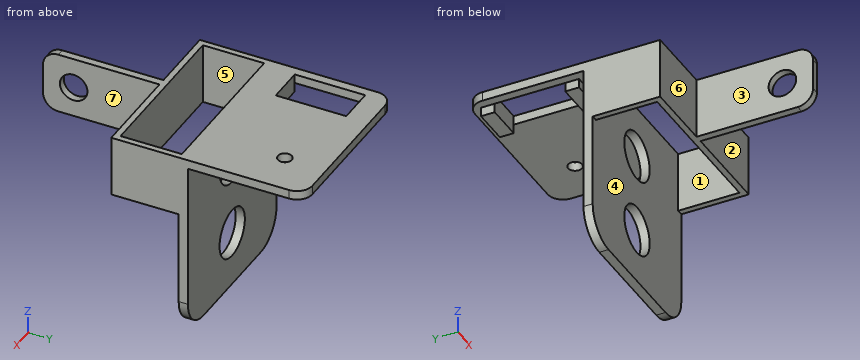
from build123d import *

# Parameters (mm, degrees)
SKETCH1_W                = 50
SKETCH1_H                = 57.8
BOSS_EXTRUDE1_DEPTH      = 3
SKETCH1_3_W              = 50
SKETCH1_3_H              = 3
BOSS_EXTRUDE2_DEPTH      = 63
SKETCH7_W                = 10
SKETCH7_H                = 20
BOSS_EXTRUDE6_DEPTH      = 60
SKETCH8_W                = 7.5
SKETCH8_H                = 20
CUT_EXTRUDE4_DEPTH       = 60
SKETCH10_R               = 4.5
CUT_EXTRUDE5_DEPTH       = 60
FILLET1_R                = 5
FILLET2_R                = 5
CUT_EXTRUDE6_REACH       = 93.771
FILLET4_R                = 5
BOSS_EXTRUDE7_DEPTH      = 3
BOSS_EXTRUDE8_DEPTH      = 3
SKETCH15_R               = 8
CUT_EXTRUDE7_DEPTH       = 3
CUT_EXTRUDE8_DEPTH       = 40
BOSS_EXTRUDE9_DEPTH      = 23
BOSS_EXTRUDE9_DEPTH_BACK = 33
SKETCH17_W               = 20
SKETCH17_H               = 2
BOSS_EXTRUDE25_REACH     = 95.87
SKETCH19_W               = 54
SKETCH19_H               = 20
SKETCH19_W_2             = 2
CUT_EXTRUDE9_REACH       = 83.018
CUT_EXTRUDE10_REACH      = 78.756
SKETCH27_R               = 8
SKETCH28_W               = 12
SKETCH28_H               = 4.5
BOSS_EXTRUDE26_DEPTH     = 3
SKETCH28_3_W             = 12
SKETCH28_3_H             = 23
CUT_EXTRUDE11_DEPTH      = 3
SKETCH29_W               = 56
SKETCH29_H               = 22
CUT_EXTRUDE12_DEPTH      = 3
FILLET5_R                = 5
FILLET6_R                = 10
CUT_EXTRUDE13_REACH      = 90.719
SKETCH30_R               = 2.271159968


with BuildPart() as part:
    # Sketch1 → Boss-Extrude1 (new body)
    with BuildSketch(Plane(origin=(0, 0, 0), x_dir=(1, 0, 0), z_dir=(0, 1, 0))):
        with Locations((2.5, 0.4)):
            Rectangle(SKETCH1_W, SKETCH1_H)
    extrude(amount=BOSS_EXTRUDE1_DEPTH)

    # Sketch1<3> → Boss-Extrude2 (add)
    with BuildSketch(Plane(origin=(0, 0, 0), x_dir=(1, 0, 0), z_dir=(0, 1, 0))):
        with Locations((2.5, -30)):
            Rectangle(SKETCH1_3_W, SKETCH1_3_H)
    extrude(amount=BOSS_EXTRUDE2_DEPTH)

    # Sketch7 → Boss-Extrude6 (add)
    with BuildSketch(Plane.XZ):
        with Locations((2.5, 21.5)):
            Rectangle(SKETCH7_W, SKETCH7_H)
    extrude(amount=BOSS_EXTRUDE6_DEPTH)

    # Sketch8 → Cut-Extrude4 (cut)
    with BuildSketch(Plane(origin=(0, 0, 11.5), x_dir=(-1, 0, 0), z_dir=(0, 0, -1))):
        with Locations((-3.75, -50)):
            Rectangle(SKETCH8_W, SKETCH8_H)
    extrude(amount=-CUT_EXTRUDE4_DEPTH, mode=Mode.SUBTRACT)

    # Sketch10 → Cut-Extrude5 (cut)
    with BuildSketch(Plane(origin=(0, 0, 0), x_dir=(0, 0, -1), z_dir=(1, 0, 0))):
        with Locations((-21.5, -50)):
            Circle(SKETCH10_R)
    extrude(amount=-CUT_EXTRUDE5_DEPTH, mode=Mode.SUBTRACT)

    # Fillet1
    fillet1_edges = [part.edges().sort_by_distance(p)[0] for p in [
        (7.5, -20, 11.5),
    ]]
    fillet(fillet1_edges, radius=FILLET1_R)

    # Fillet2
    fillet2_edges = [part.edges().sort_by_distance(p)[0] for p in [
        (7.5, -20, 31.5),
    ]]
    fillet(fillet2_edges, radius=FILLET2_R)

    # Sketch11 → Cut-Extrude6 (cut, up to next)
    with BuildSketch(Plane.XY.offset(31.5), mode=Mode.PRIVATE) as cut_extrude6_sk1:
        with BuildLine():
            Line((7.5, -40), (0, -40))
            Line((0, -40), (0, -20))
            ThreePointArc((0, -20), (2.621852946, -15.723111223), (7.5, -14.552824164))
            Line((7.5, -14.552824164), (7.5, -40))
        make_face()
    cut_extrude6_tool1 = extrude(cut_extrude6_sk1.sketch, amount=-CUT_EXTRUDE6_REACH, mode=Mode.PRIVATE) & part.part
    add(cut_extrude6_tool1.solids().sort_by_distance((3.859065, -27.782641, 31.5))[0], mode=Mode.SUBTRACT)

    # Fillet4
    fillet4_edges = [part.edges().sort_by_distance(p)[0] for p in [
        (-1.25, -60, 11.5),
        (-1.25, -60, 31.5),
    ]]
    fillet(fillet4_edges, radius=FILLET4_R)

    # Sketch13 → Boss-Extrude7 (add)
    with BuildSketch(Plane(origin=(27.5, 0, 0), x_dir=(0, 0, -1), z_dir=(1, 0, 0))):
        Polygon((-31.5, 0), (29.3, 0), (29.3, 3), (-28.5, 3), (-28.5, 63), (-31.5, 63), align=None)
    extrude(amount=BOSS_EXTRUDE7_DEPTH)

    # Sketch14 → Boss-Extrude8 (add)
    with BuildSketch(Plane.ZY.offset(22.5)):
        Polygon((-29.3, 0), (31.5, 0), (31.5, 63), (28.5, 63), (28.5, 3), (-29.3, 3), align=None)
    extrude(amount=BOSS_EXTRUDE8_DEPTH)

    # Sketch15 → Cut-Extrude7 (cut)
    with BuildSketch(Plane(origin=(0, 3, 0), x_dir=(1, 0, 0), z_dir=(0, 1, 0))):
        with Locations(Location((2.5, 11.3, 0), (0, 0, 270))):
            Circle(SKETCH15_R)
        with Locations(Location((2.5, -14.7, 0), (0, 0, 270))):
            Circle(SKETCH15_R)
    extrude(amount=-CUT_EXTRUDE7_DEPTH, mode=Mode.SUBTRACT)

    # Sketch16 → Cut-Extrude8 (cut, symmetric)
    with BuildSketch(Plane(origin=(0, 0, 0), x_dir=(0, 0, -1), z_dir=(1, 0, 0))):
        Polygon((-31.5, -20), (-11.5, -20), (-11.5, 0), (-31.5, 0.262000387), align=None)
    extrude(amount=CUT_EXTRUDE8_DEPTH, both=True, mode=Mode.SUBTRACT)


with BuildPart() as cut_extrude8_piece_1:
    # of the separate pieces the step leaves, piece 1, a body of its own (cut_extrude8_pieces)
    add(part.part.solids().sort_by_distance((30.5, 63, 31.5))[0])



with BuildPart() as cut_extrude8_piece_2:
    # of the separate pieces the step leaves, piece 2, a body of its own (cut_extrude8_pieces)
    add(part.part.solids().sort_by_distance((0, -55, 31.5))[0])

    # Sketch17 → Boss-Extrude9 (add, two sides: drawn at the far end of the back side and taken through both)
    with BuildSketch(Plane.ZY.offset(2.5).offset(-BOSS_EXTRUDE9_DEPTH_BACK)):
        with Locations((21.5, -21)):
            Rectangle(SKETCH17_W, SKETCH17_H)
    extrude(amount=BOSS_EXTRUDE9_DEPTH + BOSS_EXTRUDE9_DEPTH_BACK)


with BuildPart() as cut_extrude8_piece_1_1:
    add(cut_extrude8_piece_1.part)

    add(cut_extrude8_piece_2.part)  # Boss-Extrude25 merges Cut-Extrude8 piece 2
    # Boss-Extrude25: up to this plane
    boss_extrude25_end = Plane(origin=(-40, 0, 11.5), z_dir=(0, 0.9999142057885084, -0.013098895462462855))
    # Sketch19 → Boss-Extrude25 (add, up to the surface)
    with BuildSketch(Plane(origin=(0, -20, 0), x_dir=(1, 0, 0), z_dir=(0, 1, 0)), mode=Mode.PRIVATE) as boss_extrude25_sk1:
        with Locations((1.5, -21.5)):
            Rectangle(SKETCH19_W, SKETCH19_H)
    boss_extrude25_tool1 = split(extrude(boss_extrude25_sk1.sketch, amount=BOSS_EXTRUDE25_REACH, mode=Mode.PRIVATE), bisect_by=boss_extrude25_end, keep=Keep.BOTH, mode=Mode.PRIVATE)
    add(boss_extrude25_tool1.solids().sort_by_distance((1.5, -20, 21.5))[0])
    # Sketch19 → Boss-Extrude25 (add, up to the surface)
    with BuildSketch(Plane(origin=(0, -20, 0), x_dir=(1, 0, 0), z_dir=(0, 1, 0)), mode=Mode.PRIVATE) as boss_extrude25_sk2:
        with Locations((29.5, -21.5)):
            Rectangle(SKETCH19_W_2, SKETCH19_H)
    boss_extrude25_tool2 = split(extrude(boss_extrude25_sk2.sketch, amount=BOSS_EXTRUDE25_REACH, mode=Mode.PRIVATE), bisect_by=boss_extrude25_end, keep=Keep.BOTH, mode=Mode.PRIVATE)
    add(boss_extrude25_tool2.solids().sort_by_distance((29.5, -20, 21.5))[0])

    # Sketch25 → Cut-Extrude9 (cut, up to next)
    with BuildSketch(Plane(origin=(0, 0, 11.5), x_dir=(-1, 0, 0), z_dir=(0, 0, -1)), mode=Mode.PRIVATE) as cut_extrude9_sk1:
        Polygon((-9.832121112, 0), (-28.5, 0), (-28.5, -20), (23.5, -20), (23.5, 0), (4.832121112, 0), align=None)
    cut_extrude9_tool1 = extrude(cut_extrude9_sk1.sketch, amount=-CUT_EXTRUDE9_REACH, mode=Mode.PRIVATE) & cut_extrude8_piece_1_1.part
    add(cut_extrude9_tool1.solids().sort_by_distance((2.5, -10, 11.5))[0], mode=Mode.SUBTRACT)

    # Sketch27 → Cut-Extrude10 (cut, up to next)
    with BuildSketch(Plane.XZ, mode=Mode.PRIVATE) as cut_extrude10_sk1:
        with Locations(Location((2.5, 14.7, 0), (0, 0, 90))):
            Circle(SKETCH27_R)
    cut_extrude10_tool1 = extrude(cut_extrude10_sk1.sketch, amount=-CUT_EXTRUDE10_REACH, mode=Mode.PRIVATE) & cut_extrude8_piece_1_1.part
    add(cut_extrude10_tool1.solids().sort_by_distance((2.5, 0, 14.7))[0], mode=Mode.SUBTRACT)

    # Sketch28 → Boss-Extrude26 (add)
    with BuildSketch(Plane(origin=(0, 0, 28.5), x_dir=(-1, 0, 0), z_dir=(0, 0, -1))):
        with Locations((16.5, 35.75)):
            Rectangle(SKETCH28_W, SKETCH28_H)
        with Locations((16.5, 8.25)):
            Rectangle(SKETCH28_W, SKETCH28_H)
    extrude(amount=BOSS_EXTRUDE26_DEPTH)

    # Sketch28<3> → Cut-Extrude11 (cut)
    with BuildSketch(Plane(origin=(0, 0, 28.5), x_dir=(-1, 0, 0), z_dir=(0, 0, -1))):
        with Locations((16.5, 22)):
            Rectangle(SKETCH28_3_W, SKETCH28_3_H)
    extrude(amount=-CUT_EXTRUDE11_DEPTH, mode=Mode.SUBTRACT)

    # Sketch29 → Cut-Extrude12 (cut)
    with BuildSketch(Plane(origin=(0, 0, 28.5), x_dir=(-1, 0, 0), z_dir=(0, 0, -1))):
        with Locations((-2.5, 52)):
            Rectangle(SKETCH29_W, SKETCH29_H)
    extrude(amount=-CUT_EXTRUDE12_DEPTH, mode=Mode.SUBTRACT)

    # Fillet5
    fillet5_edges = [cut_extrude8_piece_1_1.edges().sort_by_distance(p)[0] for p in [
        (-25.5, 41, 30),
        (30.5, 41, 30),
    ]]
    fillet(fillet5_edges, radius=FILLET5_R)

    # Fillet6
    fillet6_edges = [cut_extrude8_piece_1_1.edges().sort_by_distance(p)[0] for p in [
        (30.5, 1.5, -29.3),
        (-25.5, 1.5, -29.3),
    ]]
    fillet(fillet6_edges, radius=FILLET6_R)

    # Sketch30 → Cut-Extrude13 (cut, up to next)
    with BuildSketch(Plane(origin=(0, 0, 28.5), x_dir=(-1, 0, 0), z_dir=(0, 0, -1)), mode=Mode.PRIVATE) as cut_extrude13_sk1:
        with Locations((-16.5, 27.4)):
            Circle(SKETCH30_R)
    cut_extrude13_tool1 = extrude(cut_extrude13_sk1.sketch, amount=-CUT_EXTRUDE13_REACH, mode=Mode.PRIVATE) & cut_extrude8_piece_1_1.part
    add(cut_extrude13_tool1.solids().sort_by_distance((16.5, 27.4, 28.5))[0], mode=Mode.SUBTRACT)


solid = cut_extrude8_piece_1_1.part
Geometry: final body of the model. Coordinates: model frame, mm. Face numbers are marked on the shaded views. A direction names the side the tool comes from. Give positions to 0.01 mm unless a question says otherwise; leave off trailing zeros. Loops run counter-clockwise (first coordinate to the right, second up) from the corner with the lowest first, then second, coordinate; pieces in that order, holes last. Notation, with made-up numbers: (27, 62.25) - (38, 62.25) arc R34 cw to (38, 101.25) - close; hole circle Ø9 at (68.5, -25.5). An arc over 180 degrees is marked (long way). One line per question, with ' | ' between items. Start each with the question number.
(1) Section query D-D on x = 16.5. Return loops of the section in (y, z).
(2) Section query B-B on x = -7. Return loops of the section in (y, z).
(3) Reachability of the marked faces 5, 6 and 7 from +Z, -Z, +X, -X, +Y, -Y: full face, straight path, thin tool, end or side. Return the list, or none.
(4) Contact query for flat-ended pins moving along their axis: pin 1 (11.5 mm diameter, centred on x = 5, y = 25, fed in from -Z); pin 2 (4 mm diameter, centred on x = 15.5, z = -9, fed in from -Y); pin 3 (6 mm diameter, centred on y = -44, z = 24, fed in from -X); pin 4 (3.5 mm diameter, centred on x = -15.5, z = 27.5, fed in from +Y). Output: stop coordinate, or through.
(5) Section query C-C on y = -50. Return loops of the section in (x, z).
(6) Pull-direction query (Y, two-part tool) for the marked faces 1, 2, 3 and 4; classes: released by +Y, released by -Y, zero draft, split by the parting line, or undercut.
(7) Section query A-A on z = -5.5. Return loops of the section in (x, y), then the cut area to 3 significant figures.
(8) Ray query, line 1 (X direction, y = 2.15, z = -11.3); line 2 (X direction, y = 27, z = 29); line 3 (Y direction, x = -12, z = 23.5). Return the intervals inside material, ascending. Write a range as from..to.
The answers:
1) outline: (-22, 11.5) - (-20, 11.5) - (-20, 31.5) - (-22, 31.5) - close; (0, -29.3) - (3, -29.3) - (3, 28.5) - (25.13, 28.5) - (25.13, 31.5) - (0, 31.5) - close; (29.67, 28.5) - (41, 28.5) - (41, 31.5) - (29.67, 31.5) - close
2) outline: (-22, 11.5) - (-20, 11.5) - (-20, 31.5) - (-22, 31.5) - close; (0, -29.3) - (3, -29.3) - (3, 28.5) - (41, 28.5) - (41, 31.5) - (0, 31.5) - close
3) face 5: +Z, -Z | face 6: +Z, -Z, -X, -Y | face 7: +Z, -Z, +X, -Y
4) pin 1: z = 28.5 | pin 2: y = 0 | pin 3: x = -2.5 | pin 4: y = 41
5) outline: (-2.5, 11.5) - (0, 11.5) - (0, 17) - (-2.5, 17) - close; (-2.5, 26) - (0, 26) - (0, 31.5) - (-2.5, 31.5) - close
6) face 1: undercut | face 2: released by -Y | face 3: zero draft | face 4: undercut
7) outline: (-25.5, 0) - (-3.01, 0) - (-3.01, 3) - (-25.5, 3) - close; (8.01, 0) - (30.5, 0) - (30.5, 3) - (8.01, 3) - close | area: 135 mm2
8) line 1: -25.5..-5.5, 10.5..30.5 | line 2: -25.5..-22.5, -10.5..14.26, 18.74..30.5 | line 3: -22..-20, 0..3
